```python
from build123d import *

# Parameters (mm, degrees)
F0_R     = 1.5875
F1_DEPTH = 3.175


# Not quite as in the source:
# - ends of sketch curves that miss each other by under 0.0002 mm in the source are joined
# - a feature names something its author has since deleted; it is built from what else it names


with BuildPart() as f1:
    # F0 (on Front) → F1 (new body)
    with BuildSketch(Plane.XZ):
        with BuildLine():
            Line((8.7026358494, -4.754912237), (7.4606623464, -3.512938734))
            ThreePointArc((7.4606623464, -3.512938734), (8.3275358886, -4.9102837361), (8.7026358494, -6.5113280243))
            Line((8.7026358494, -6.5113280243), (8.7026358494, -4.754912237))
        make_face()
        with BuildLine():
            Line((-10.3241423466, 14.271865959), (-11.6173641506, 15.565087763))
            Line((-11.6173641506, 15.565087763), (-13.4462559649, 15.565087763))
            ThreePointArc((-13.4462559649, 15.565087763), (-11.774512383, 15.185698369), (-10.3241423466, 14.271865959))
        make_face()
        with BuildLine():
            ThreePointArc((-8.0252617022, 19.1571902114), (-9.6733323142, 20.2583957881), (-11.6173641506, 20.645087763))
            Line((-11.6173641506, 20.645087763), (-11.6173641506, 15.565087763))
            Line((-11.6173641506, 15.565087763), (-8.0252617022, 19.1571902114))
        make_face()
        with BuildLine():
            ThreePointArc((13.7826358494, -4.7549120495), (13.3959438387, -2.810880314), (12.2947382978, -1.1628097886))
            Line((12.2947382978, -1.1628097886), (8.7026358494, -4.754912237))
            Line((8.7026358494, -4.754912237), (9.4338794152, -4.75491221))
            ThreePointArc((9.4338794152, -4.75491221), (11.0213794287, -3.167412237), (12.6088794152, -4.754912237))
            Line((12.6088794152, -4.754912237), (13.7826358494, -4.7549120495))
        make_face()
        with BuildLine():
            ThreePointArc((-34.4773641506, 20.645087763), (-36.2734153748, 19.9011389872), (-37.0173641506, 18.105087763))
            Line((-37.0173641506, 18.105087763), (-37.0173641506, -4.754912237))
            ThreePointArc((-37.0173641506, -4.754912237), (-34.4773641506, -7.294912237), (-31.9373641506, -4.754912237))
            Line((-31.9373641506, -4.754912237), (-31.9373641506, 13.025087763))
            Line((-31.9373641506, 13.025087763), (-31.9373641506, 15.565087763))
            Line((-31.9373641506, 15.565087763), (-31.9373641506, 20.645087763))
            Line((-31.9373641506, 20.645087763), (-34.4773641506, 20.645087763))
        make_face()
        with Locations((-34.4773641506, -4.754912237)):
            Circle(F0_R, mode=Mode.SUBTRACT)
        Polygon((-11.6173641506, 20.645087763), (-31.9373641506, 20.645087763), (-31.9373641506, 15.565087763), (-29.3973641506, 15.565087763), (-13.4462559649, 15.565087763), (-11.6173641506, 15.565087763), align=None)
        with BuildLine():
            ThreePointArc((11.2426358494, -30.154912237), (13.0386870736, -29.4109634612), (13.7826358494, -27.614912237))
            Line((13.7826358494, -27.614912237), (12.8301358494, -27.614912237))
            ThreePointArc((12.8301358494, -27.614912237), (11.2426358494, -29.202412237), (9.6551358494, -27.614912237))
            Line((9.6551358494, -27.614912237), (8.7026358494, -27.614912237))
            ThreePointArc((8.7026358494, -27.614912237), (9.4465846252, -29.4109634612), (11.2426358494, -30.154912237))
        make_face()
        with BuildLine():
            Line((9.4338794152, -4.75491221), (8.7026358494, -4.754912237))
            Line((8.7026358494, -4.754912237), (8.7026358494, -6.5113280243))
            Line((8.7026358494, -6.5113280243), (8.7026358494, -27.614912237))
            Line((8.7026358494, -27.614912237), (9.6551358494, -27.614912237))
            ThreePointArc((9.6551358494, -27.614912237), (11.2426358494, -26.027412237), (12.8301358494, -27.614912237))
            Line((12.8301358494, -27.614912237), (13.7826358494, -27.614912237))
            Line((13.7826358494, -27.614912237), (13.7826358494, -4.7549120495))
            Line((13.7826358494, -4.7549120495), (12.6088794152, -4.7549120928))
            ThreePointArc((12.6088794152, -4.7549120928), (11.0213794017, -6.342412237), (9.4338794152, -4.75491221))
        make_face()
        Polygon((-8.0252617022, 19.1571902114), (-11.6173641506, 15.565087763), (-10.3241423466, 14.271865959), (7.4606623464, -3.512938734), (8.7026358494, -4.754912237), (12.2947382978, -1.1628097886), align=None)
    extrude(amount=F1_DEPTH)


solid = f1.part
```
The listing builds one solid part. Answer for the finished solid, in the listing's coordinates (mm). A direction names the side the tool comes from. Give positions to 0.01 mm unless a question says otherwise; leave off trailing zeros. Order: outer loops, then holes, each group sorted by start corner. A loop starts at its lowest first (then second) coordinate and runs counter-clockwise, first axis right, second up.
1) Find section B-B on z = -0.5. Write down the section's boundary in (x, y) (3 decimals).
Reported:
outline: (-37.017, -3.175) - (-31.937, -3.175) - (-31.937, 0) - (-37.017, 0) - close; (4.448, -3.175) - (11.632, -3.175) - (11.632, 0) - (4.448, 0) - close
2) Find section C-C on x = -30.5. Write down the section's boundary in (y, z) (3 decimals), then the cut area to 3 significant figures.
Reported:
outline: (-3.175, 15.565) - (0, 15.565) - (0, 20.645) - (-3.175, 20.645) - close
area: 16.1 mm2
3) Consider line 1 along Z through (x, y) = (-17, -2.25); line 2 along X through (y, z) = (-0.25, -11.5); line 3 along X through (y, z) = (-2.3, 11). Determine where each line is inside the solid, lowest interval first.
Reported:
line 1: z = 15.57 to 20.65
line 2: x = 8.7 to 13.78
line 3: x = -37.02 to -31.94, -7.05 to 0.13
4) Find section A-A on y = -2.3. Write down the section's boundary in (x, z) (1 decimal).
Reported:
outline: (-37, -4.8) arc R2.5 ccw to (-31.9, -4.8) - (-31.9, 15.6) - (-13.4, 15.6) arc R5.1 cw to (-10.3, 14.3) - (7.5, -3.5) arc R5.1 cw to (8.7, -6.5) - (8.7, -27.6) arc R2.5 ccw to (13.8, -27.6) - (13.8, -4.8) arc R5.1 ccw to (12.3, -1.2) - (-8, 19.2) arc R5.1 ccw to (-11.6, 20.6) - (-34.5, 20.6) arc R2.5 ccw to (-37, 18.1) - close; hole circle Ø3.2 at (-34.5, -4.8); hole circle Ø3.2 at (11, -4.8); hole circle Ø3.2 at (11.2, -27.6)
5) Find section D-D on z = -17. Write down the section's boundary in (x, y) (3 decimals), then the cut area to 3 significant figures.
Reported:
outline: (8.703, -3.175) - (13.783, -3.175) - (13.783, 0) - (8.703, 0) - close
area: 16.1 mm2
6) Given P1, Ø1.6, axis at x = -22.5, y = -1, coming from the -Z side, flat-ended and moving along its own axis, determine where the tip first touches the part or whether it passes through.
Reported:
P1: stops at z = 15.57
7) Determine the mould class of faces 1 (the face through (8.703, -2, -17)), 2 (the face through (-9.65, -1.57, 20.25)), 3 (the face through (-32.963, -1.565, -4.278)), 4 (the face through (11.98, -1.57, -26.21)) for opening direction Z: pulls with the +Z half, pulls with the -Z half, needs draft (parallel to the pull), parting line crosses it, or undercut.
Reported:
face 1: needs draft
face 2: pulls with the +Z half
face 3: undercut
face 4: undercut
8) For faces 5 (the face through (-11.797, -1.565, 15.195)), 6 (the face through (-36.254, -1.565, 19.921)), determine the directions among +Z, -Z, +X, -X, +Y, -Y from which every point of the face is accessible in a straight line to the end or side of a thin tool.
Reported:
face 5: -Z, +Y, -Y
face 6: +Z, -X, +Y, -Y
